```python
from build123d import *

# Parameters (mm, degrees)
F1_DEPTH = 50.8
F2_R     = 2.54
F3_DEPTH = 25.4


with BuildPart() as f1:
    # F0 (on Right) → F1 (new body)
    with BuildSketch(Plane.YZ):
        Polygon((-19.05, 0), (0, 0), (0, 25.4), (-3.175, 25.4), (-3.175, 3.175), (-19.05, 3.175), align=None)
    extrude(amount=F1_DEPTH)

    # F2 (on Front) → F3 (cut)
    with BuildSketch(Plane.XZ):
        with Locations((38.1, 12.7)):
            Circle(F2_R)
        with Locations((12.7, 12.7)):
            Circle(F2_R)
    extrude(amount=F3_DEPTH, mode=Mode.SUBTRACT)


solid = f1.part
```
CAD build for the part. Positions are in the model's coordinates, mm. A direction names the side the tool comes from. Coordinates: 2 decimals unless noted, no trailing zeros. Order: outer loops, then holes, each group sorted by start corner. A loop starts at its lowest first (then second) coordinate and runs counter-clockwise, first axis right, second up. Notation, with made-up numbers: M 46,34.5 L 67,34.5 A7 ccw 67,41.5 Z; hole C 32.25,3 d7. An arc over 180 degrees is marked long. Write each question's results on one line, items separated by ' | '. Start each with the question number.
Q1. Cut at D-D (y = -11). List the corners of the cut face in (x, z) (3 decimals), then the cut area to 3 significant figures.
Q2. Cut at B-B (z = 12.7). List the corners of the cut face in (x, y) (3 decimals).
Q3. Drill centre lines: probe 1 along X at (y, z) = (-2.4, 12.7); probe 2 along Z at (x, y) = (12.7, -1.35); probe 3 along Y at (x, z) = (43.5, 20.25) (3 decimals). Where is each one in solid material? Low to high. Write a range as from..to.
Q4. Pull direction Z, two halves, no side cores. Call faces 3 (the flat face through (25, -10, 0)), 4 (the flat face through (25, -3.175, 14)), 5 (the cylindrical face through (35.562, -1.565, 12.812)), 6 (the flat face through (25, -2, 25.4)): +Z half, -Z half, draft (parallel to the pull), parting line (faces both ways), or undercut.
Q5. Which spindle directions (+Z, -Z, +X, -X, +Y, -Y) get a long thin tool onto all of the face, cutting with end or side? Do faces 1 (the flat face through (0, -3, 8)), 2 (the flat face through (25, -11, 3.175)). Say none if no direction does.
Q6. Flat gauge pins, fed straight in: P1, Ø5, axis at x = 17, y = -11.5, coming from the +Z side (3 decimals); P2, Ø12, axis at x = 20.5, z = 14.5, coming from the -Y side (3 decimals). Where does each tip first touch, or does it go through?
Q7. Cut at A-A (x = 38.1). List the corners of the cut face in (y, z) (3 decimals), then the cut area to 3 significant figures.
Q8. Cut at C-C (x = 29). List the corners of the cut face in (y, z) (3 decimals).
Found:
1) outline: M 0,0 L 50.8,0 L 50.8,3.175 L 0,3.175 Z | area: 161 mm²
2) outline: M 0,-3.175 L 10.16,-3.175 L 10.16,0 L 0,0 Z; M 15.24,-3.175 L 35.56,-3.175 L 35.56,0 L 15.24,0 Z; M 40.64,-3.175 L 50.8,-3.175 L 50.8,0 L 40.64,0 Z
3) probe 1: 0..10.16, 15.24..35.56, 40.64..50.8 | probe 2: 0..10.16, 15.24..25.4 | probe 3: -3.175..0
4) face 3: -Z half | face 4: draft | face 5: undercut | face 6: +Z half
5) face 1: +Z, -Z, -X, +Y, -Y | face 2: +Z, +X, -X, -Y
6) P1: z = 3.175 | P2: y = -3.175
7) outline: M -19.05,0 L 0,0 L 0,10.16 L -3.175,10.16 L -3.175,3.175 L -19.05,3.175 Z; M -3.175,15.24 L 0,15.24 L 0,25.4 L -3.175,25.4 Z | area: 115 mm²
8) outline: M -19.05,0 L 0,0 L 0,25.4 L -3.175,25.4 L -3.175,3.175 L -19.05,3.175 Z
